For this review, take the finished solid that the model builds, in its own axes (mm). Face numbers are marked on the shaded views. A direction names the side the tool comes from. Give positions to 0.01 mm unless a question says otherwise; leave off trailing zeros. Loops run counter-clockwise (first coordinate to the right, second up) from the corner with the lowest first, then second, coordinate; pieces in that order, holes last. Notation, with made-up numbers: (-21, 48) -> (16, 48) arc R24 ccw to (16, 76) -> close; hole circle Ø11 at (25.5, -20). An arc over 180 degrees is marked (long way). One line per question, with ' | ' between items. Start each with the question number.
(1) Consider section A-A (z = 0). Write out the cut boundary in (x, y), and give its area (3 significant figures).
(2) Consider section D-D (x = 6.75). Write out the cut boundary in (y, z), and give its area (3 significant figures).
(3) Wall thickness on probe 1 along Y at (x, z) = (6.75, -4); probe 2 along Z at (x, y) = (0, 6): over which ranges is each line inside the solid? List them lowest first.
(4) Insertion check: P1, Ø5, axis at x = 2.5, y = 7.5, coming from the +Z side; P2, Ø1.5, axis at x = -1, z = 1, coming from the +Y side; P3, Ø1.5, axis at y = 6, z = 5, coming from the +X side; P4, Ø3, axis at y = 10, z = 5.5, coming from the +X side. Each pin has a flat end and moves straight along its axis. Give the tip position at first contact, or say it passes through.
(5) Consider section B-B (x = 0). Write out the cut boundary in (y, z).
(6) Tool access review of the marked faces 5 and 6: name each direction out of +Z, -Z, +X, -X, +Y, -Y from which nothing blocks a thin tool from reaching the whole face with its end or side.
(7) Draft analysis for pull direction Y (two halves, no side actions). For the marked faces 1, 2, 3 and 4, state which applies: +Y half, -Y half, draft (parallel to the pull), parting line (faces both ways), or undercut.
(8) Consider section C-C (y = 4.25). Write out the cut boundary in (x, z).
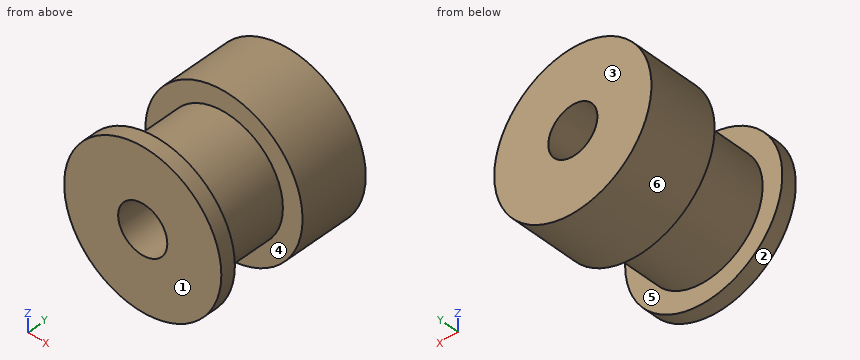
from build123d import *

# Parameters (mm, degrees)
SKETCH1_R           = 8
SKETCH1_R_2         = 2.5
BOSS_EXTRUDE1_DEPTH = 16
CUT_EXTRUDE1_START  = -7
SKETCH2_R           = 8
SKETCH2_R_2         = 6
CUT_EXTRUDE1_DEPTH  = 7.5


with BuildPart() as part:
    # Sketch1 → Boss-Extrude1 (new body)
    with BuildSketch(Plane(origin=(0, 0, 0), x_dir=(1, 0, 0), z_dir=(0, 1, 0))):
        Circle(SKETCH1_R)
        Circle(SKETCH1_R_2, mode=Mode.SUBTRACT)
    extrude(amount=BOSS_EXTRUDE1_DEPTH)

    # Sketch2 → Cut-Extrude1 (cut)
    with BuildSketch(Plane(origin=(0, 16, 0), x_dir=(1, 0, 0), z_dir=(0, 1, 0)).offset(CUT_EXTRUDE1_START)):
        Circle(SKETCH2_R)
        Circle(SKETCH2_R_2, mode=Mode.SUBTRACT)
    extrude(amount=-CUT_EXTRUDE1_DEPTH, mode=Mode.SUBTRACT)


solid = part.part
A:
1) outline: (-8, 0) -> (-2.5, 0) -> (-2.5, 16) -> (-8, 16) -> (-8, 9) -> (-6, 9) -> (-6, 1.5) -> (-8, 1.5) -> close; (2.5, 0) -> (8, 0) -> (8, 1.5) -> (6, 1.5) -> (6, 9) -> (8, 9) -> (8, 16) -> (2.5, 16) -> close | area: 146 mm^2
2) outline: (0, -4.29) -> (1.5, -4.29) -> (1.5, 4.29) -> (0, 4.29) -> close; (9, -4.29) -> (16, -4.29) -> (16, 4.29) -> (9, 4.29) -> close | area: 73.0 mm^2
3) probe 1: y = 0 to 1.5, 9 to 16 | probe 2: z = -6 to -2.5, 2.5 to 6
4) P1: stops at z = 7.98 | P2: passes through | P3: stops at x = 4.24 | P4: stops at x = 6.93
5) outline: (0, -8) -> (1.5, -8) -> (1.5, -6) -> (9, -6) -> (9, -8) -> (16, -8) -> (16, -2.5) -> (0, -2.5) -> close; (0, 2.5) -> (16, 2.5) -> (16, 8) -> (9, 8) -> (9, 6) -> (1.5, 6) -> (1.5, 8) -> (0, 8) -> close
6) face 5: none | face 6: +Y, -Y
7) face 1: -Y half | face 2: draft | face 3: +Y half | face 4: undercut
8) outline: circle Ø12 at (0, 0); hole circle Ø5 at (0, 0)
